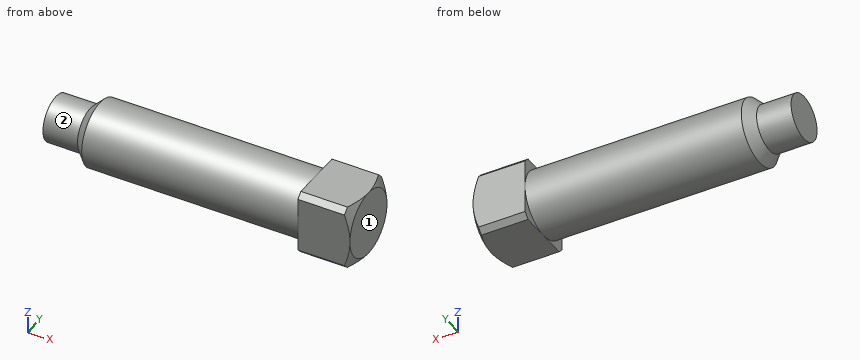
Autodesk Inventor part; units mm, degrees
ref_plane "Work Plane1" through (0, 0, 0) normal (0, 0, 1) x (1, 0, 0)
ref_plane "YZ Plane" through (0, 0, 0) normal (1, 0, 0) x (0, 1, 0)
ref_plane "XZ Plane" through (0, 0, 0) normal (0, 1, 0) x (-1, 0, 0)
sketch "Эскиз1" plane through (0, 0, 0) normal (0, 0, 1) x (1, 0, 0)
  line L0 (40, 0) -> (40, 5)
  line L1 (40, 5) -> (5.3, 5)
  line L2 (40, 0) -> (0, 0)
  line L3 (5.3, 3.5) -> (0, 3.5)
  line L4 (0, 3.5) -> (0, 0)
  line L5 (5.3, 5) -> (5.3, 3.5)
  line L6 (0, 6) -> (0, -1)
  line L7 (-8, 0) -> (48, 0)
  dimension "d0" = 10
  dimension "d10" = 40
  dimension "d11" = 7
  dimension "d12" = 5.3
revolve "Базовый элемент" add sketch "Эскиз1" angle 360 about axis through (40, 0, 0) along (-1, 0, 0)
sketch "Эскиз2" plane through (40, 0, 0) normal (1, 0, 0) x (0, 0, -1)
  line L0 (0, 5) -> (4.1924, 5)
  line L1 (5, 4.1924) -> (5, 0)
  line L2 (5, 0) -> (0, 0) construction
  line L3 (0, 0) -> (0, 5) construction
  line L4 (0, -7) -> (0, 7)
  line L5 (7, 0) -> (-7, 0)
  line L6 (0, 5) -> (-4.1924, 5)
  line L7 (-5, 4.1924) -> (-5, -4.1924)
  line L8 (0, -5) -> (4.1924, -5)
  line L9 (5, -4.1924) -> (5, 0)
  line L10 (0, -5) -> (-4.1924, -5)
  line L11 (-5, -4.1924) -> (-5, 0)
  circle A0 centre (0, 0) radius 5
  line L12 (4.1924, 5) -> (5, 4.1924)
  line L13 (5, -4.1924) -> (4.1924, -5)
  line L14 (-4.1924, -5) -> (-5, -4.1924)
  line L15 (-5, 4.1924) -> (-4.1924, 5)
  point P0 (2.0767, 5)
  point P1 (5, 2.0767)
  point P2 (-2.0767, 5)
  point P3 (-5, 2.0767)
  point P4 (2.0767, -5)
  point P5 (5, -2.0767)
  point P6 (-2.0767, -5)
  point P7 (-5, -2.0767)
  dimension "d3" = 5
  dimension "d4" = 5
  dimension "d60" = 13
extrude "С головкой" add sketch "Эскиз2" along normal blind 8
sketch "Эскиз3" plane through (0, 0, 0) normal (0, 0, 1) x (1, 0, 0)
  line L0 (48, 4.995) -> (48, 7.15)
  line L1 (48, 7.15) -> (46.8, 7.15)
  line L2 (40, 0) -> (40, 5)
  line L3 (40, 0) -> (48, 0)
  line L4 (46.8, 7.15) -> (48, 4.995)
  line L5 (0, -3.922) -> (0, 8.9953)
  line L6 (40, 5) -> (40, -2.0767)
  line L7 (48, -2.0767) -> (48, 2.0767)
  line L8 (2.4, 0) -> (55.6, 0)
  point P0 (10, -2.0767)
  point P1 (15, -2.0767)
  point P2 (15, 2.0767)
  point P3 (44, 0)
  dimension "d14" = 14.3
  dimension "d15" = 9.99
  dimension "d18" = 48
  dimension "d19" = 1.2
revolve "Фаска1" cut sketch "Эскиз3" angle 360 about axis through (40, 0, 0) along (1, 0, 0)
chamfer "Фаска2" distance 1.5 angle 45 1 edges at (5.3, -5, 0) measured on face at (16.8667, 0, -5)
thread "Резьба"
ref_plane "Work Plane1" through (0, 0, 0) normal (0, 0, 1) x (1, 0, 0)
equation "\"d0\" = NND"
equation "\"d10\" = NLG"
equation "\"d11\" = SPD"
equation "\"d12\" = ZLG"
equation "\"d3\" = 0.5 * SW"
equation "\"d4\" = 0.5 * SW"
equation "\"d60\" = KOD"
equation "\"d1\" = KOH"
equation "\"d14\" = 1.1 * KOD"
equation "\"d18\" = NLG + KOH"
equation "\"d19\" = 0.15 * KOH"
equation "\"d6\" = -0.5 * SPD + 0.5 * NND"
equation "\"d7\" = FAWI1"
equation "\"d56\" = -0.5 * SPD + 0.5 * NND"
equation "\"d16\" = NLG"
equation "\"NND\" = 10"
equation "\"NLG\" = 40"
equation "\"SPD\" = 7"
equation "\"KOD\" = 13"
equation "\"KOH\" = 8"
equation "\"FAWI1\" = 45deg"
equation "\"ZLG\" = 5.3"
equation "\"GUL\" = 0.61345 * PTC"
equation "\"TOA\" = 30deg"
equation "\"PTC\" = 1.5"
equation "\"GAL\" = 0.61345 * PTC"
equation "\"GD1\" = THREADDIA - 1.2269 * PTC"
properties part number "Винт M10-6gx40 ГОСТ 1482-84" material "Сталь, мягкая"
Check sheet for the modelled part. Datum: model origin and axes. Units: mm. Face numbers are marked on the shaded views. A direction names the side the tool comes from. Round coordinates to 2 decimals unless told otherwise and drop trailing zeros. Loops run counter-clockwise (first coordinate to the right, second up) from the corner with the lowest first, then second, coordinate; pieces in that order, holes last. Notation, with made-up numbers: M 82,25.5 L 89,25.5 A11 ccw 89,45.5 Z; hole C 84,43.5 d1. An arc over 180 degrees is marked long. One line per question, with ' | ' between items. Start each with the question number.
Item 1: Gauge pin test, flat end, axial feed: pin 1 Ø5 at (y, z) = (2.5, -3) entering from -X. Record the tip position at first contact, or that the pin passes through.
Item 2: Scan lines: probe 1 along X at (y, z) = (2.75, -3.5); probe 2 along X at (y, z) = (1, -3.5); probe 3 along Y at (x, z) = (20.5, -4.5). Record each from-to range of solid material in increasing order.
Item 3: Set-up check for the marked faces 1 and 2: record each of +Z, -Z, +X, -X, +Y, -Y from which the full face is reachable in a straight line by a thin tool's end or side.
Item 4: Section check A-A (x = 21). Record the boundary of the cut face in (y, z).
Worked out:
1) pin 1: x = 0
2) probe 1: 6.25 to 48 | probe 2: 5.44 to 48 | probe 3: -2.18 to 2.18
3) face 1: +Z, -Z, +X, +Y, -Y | face 2: -X
4) outline: C 0,0 d10
